from build123d import *

# Parameters (mm, degrees)
SKETCH1_W           = 62
SKETCH1_H           = 62
SKETCH1_R           = 10
SKETCH1_R_2         = 2
SKETCH1_R_3         = 1.5
BOSS_EXTRUDE1_DEPTH = 5
CUT_EXTRUDE2_DEPTH  = 10
SKETCH4_R           = 3
CUT_EXTRUDE3_DEPTH  = 3


with BuildPart() as part:
    # Sketch1 → Boss-Extrude1 (new body)
    with BuildSketch(Plane.XY):
        Rectangle(SKETCH1_W, SKETCH1_H)
        Circle(SKETCH1_R, mode=Mode.SUBTRACT)
        with Locations((0, 26)):
            Circle(SKETCH1_R_2, mode=Mode.SUBTRACT)
        with Locations((0, 15)):
            Circle(SKETCH1_R_3, mode=Mode.SUBTRACT)
        with Locations((22.516660498, 13)):
            Circle(SKETCH1_R_2, mode=Mode.SUBTRACT)
        with Locations((22.516660498, -13)):
            Circle(SKETCH1_R_2, mode=Mode.SUBTRACT)
        with Locations((0, -26)):
            Circle(SKETCH1_R_2, mode=Mode.SUBTRACT)
        with Locations((-22.516660498, -13)):
            Circle(SKETCH1_R_2, mode=Mode.SUBTRACT)
        with Locations((-22.516660498, 13)):
            Circle(SKETCH1_R_2, mode=Mode.SUBTRACT)
        with Locations((12.990381057, -7.5)):
            Circle(SKETCH1_R_3, mode=Mode.SUBTRACT)
        with Locations((-12.990381057, -7.5)):
            Circle(SKETCH1_R_3, mode=Mode.SUBTRACT)
    extrude(amount=BOSS_EXTRUDE1_DEPTH)

    # Sketch3 → Cut-Extrude2 (cut)
    with BuildSketch(Plane(origin=(0, 0, 0), x_dir=(-1, 0, 0), z_dir=(0, 0, -1))):
        Polygon((-31, 31), (-31, 16), (-16, 31), align=None)
        Polygon((31, 31), (16, 31), (31, 16), align=None)
        Polygon((31, -31), (31, -16), (16, -31), align=None)
        Polygon((-31, -31), (-16, -31), (-31, -16), align=None)
    extrude(amount=-CUT_EXTRUDE2_DEPTH, mode=Mode.SUBTRACT)

    # Sketch4 → Cut-Extrude3 (cut)
    with BuildSketch(Plane.XY.offset(5)):
        with Locations((0, 15)):
            Circle(SKETCH4_R)
        with Locations((12.990381057, -7.5)):
            Circle(SKETCH4_R)
        with Locations((-12.990381057, -7.5)):
            Circle(SKETCH4_R)
    extrude(amount=-CUT_EXTRUDE3_DEPTH, mode=Mode.SUBTRACT)


solid = part.part
CAD build for the part. Positions are in the model's coordinates, mm. A direction names the side the tool comes from. Coordinates: 2 decimals unless noted, no trailing zeros. Loops run counter-clockwise (first coordinate to the right, second up) from the corner with the lowest first, then second, coordinate; pieces in that order, holes last. Notation, with made-up numbers: (49.5, 89.5) - (102.5, 89.5) arc R21 cw to (102.5, 104.5) - close; hole circle Ø6 at (-33.75, 81.25). An arc over 180 degrees is marked (long way). Use one line per item in the form item = value. Start each with the question number.
1) Drill centre lines: L1, parallel to Y at x = 0, z = 3.6; L2, parallel to X at y = -8, z = 4.05; L3, parallel to X at y = -14.5, z = 2.15. Where is each one in solid material? Low to high. Write a range as from..to.
2) Band-saw the part on B-B (z = 1.2). State how many separate pieces and enclosed holes the cut face has, and give its area (3 significant figures).
3) Two-plate mould, pull along Y, no slides. Class faces 3 (the face through (-24, -23, 2)), 4 (the face through (0, 31, 2)), 5 (the face through (-0.65, 12.07, 3.52)): +Y half, -Y half, draft (parallel to the pull), parting line (faces both ways), or undercut.
4) Band-saw the part on C-C (y = -7.5). Give the cut face in (x, z).
5) Band-saw the part on A-A (y = 26). Give the cut face in (x, z), and give its area (3 significant figures).
6) Tool access for faces 1 (the face through (20.52, 13.09, 2.46)), 2 (the face through (10.78, -5.47, 3.52)): list every direction of +Z, -Z, +X, -X, +Y, -Y with a clear straight run to the whole face (end or side of a thin tool).
7) Band-saw the part on D-D (x = 17). Give the cut face in (y, z), and give its area (3 significant figures).
8) Flat gauge pin, fed straight in: pin 1 (3.5 mm diameter, centred on x = 0, y = 15, fed in from +Z). Where does the tip first touch, or does it go through?
Check values:
q1.L1 = -31..-28, -24..-10, 10..12, 18..24, 28..31
q1.L2 = -31..-15.95, -10.03..-6, 6..10.03, 15.95..31
q1.L3 = -31..-23.84, -21.19..21.19, 23.84..31
q2.separate_pieces = 1
q2.enclosed_holes = 10
q2.area = 2,980 mm2
q3.face_3 = -Y half
q3.face_4 = +Y half
q3.face_5 = undercut
q4.outline = (-31, 0) - (-14.49, 0) - (-14.49, 2) - (-15.99, 2) - (-15.99, 5) - (-31, 5) - close; (-11.49, 0) - (-6.61, 0) - (-6.61, 5) - (-9.99, 5) - (-9.99, 2) - (-11.49, 2) - close; (6.61, 0) - (11.49, 0) - (11.49, 2) - (9.99, 2) - (9.99, 5) - (6.61, 5) - close; (14.49, 0) - (31, 0) - (31, 5) - (15.99, 5) - (15.99, 2) - (14.49, 2) - close
q5.outline = (-21, 0) - (-2, 0) - (-2, 5) - (-21, 5) - close; (2, 0) - (21, 0) - (21, 5) - (2, 5) - close
q5.area = 190 mm2
q6.face_1 = +Z, -Z
q6.face_2 = +Z
q7.outline = (-30, 0) - (30, 0) - (30, 5) - (-30, 5) - close
q7.area = 300 mm2
q8.pin_1 = 2
